CAD build for the part. Positions are in the model's coordinates, mm. Face numbers are marked on the shaded views. Give positions to 0.01 mm unless a question says otherwise; leave off trailing zeros. Loops run counter-clockwise (first coordinate to the right, second up) from the corner with the lowest first, then second, coordinate; pieces in that order, holes last. Notation, with made-up numbers: M 26.5,-36 L 73.5,-36 A4 ccw 73.5,-29 Z; hole C -27.75,52.5 d10. An arc over 180 degrees is marked long. Answer as CSV lines item,"result".
from build123d import *

# Parameters (mm, degrees)
SKETCH1_R                                           = 16.5
BOSS_EXTRUDE1_DEPTH                                 = 6
SKETCH25_R                                          = 10.25
BOSS_EXTRUDE2_DEPTH                                 = 2
SKETCH22_R                                          = 2.25
CUT_EXTRUDE1_DEPTH                                  = 46.38470183
CBORE_FOR_M2_HEX_SOCKET_HEAD_CAP_SCREW1_D           = 2.4
CBORE_FOR_M2_HEX_SOCKET_HEAD_CAP_SCREW1_CBORE_D     = 4.4
CBORE_FOR_M2_HEX_SOCKET_HEAD_CAP_SCREW1_CBORE_DEPTH = 2.4
CIRPATTERN1_COUNT                                   = 4
SKETCH26_R                                          = 4.5
CUT_EXTRUDE2_DEPTH                                  = 4.5


with BuildPart() as part:
    # Sketch1 → Boss-Extrude1 (new body)
    with BuildSketch(Plane(origin=(0, 0, 0), x_dir=(1, 0, 0), z_dir=(0, 1, 0))):
        with Locations(Location((0, 0, 0), (0, 0, 270))):
            Circle(SKETCH1_R)
    extrude(amount=-BOSS_EXTRUDE1_DEPTH)

    # Sketch25 → Boss-Extrude2 (add)
    with BuildSketch(Plane.XZ.offset(6)):
        with Locations(Location((0, 0, 0), (0, 0, 270))):
            Circle(SKETCH25_R)
    extrude(amount=BOSS_EXTRUDE2_DEPTH)

    # Sketch22 → Cut-Extrude1 (cut, through all)
    with BuildSketch(Plane(origin=(1.446175283, 0, 24.410951504), x_dir=(1, 0, 0), z_dir=(0, 1, 0))):
        with Locations(Location((-1.446175283, 35.724660003, 0), (0, 0, 270))):
            Circle(SKETCH22_R)
    cut_extrude1 = extrude(amount=-CUT_EXTRUDE1_DEPTH, mode=Mode.SUBTRACT)

    # Sketch3 → Cut-Revolve1 (revolve, cut)
    with BuildSketch(Plane(origin=(0, 0, -23.450692334), x_dir=(0, 0, -1), z_dir=(1, 0, 0))):
        Polygon((-12.136983835, 0), (-8.785226394, 0), (-9.185226394, -0.4), (-9.511983835, -2.725), (-9.511983835, -5.45), (-9.886983835, -5.825), (-12.136983835, -5.825), align=None)
    cut_revolve1 = revolve(axis=Axis((0, -5.825, -11.313708499), (0, 1, 0)), mode=Mode.SUBTRACT)

    # CBORE for M2 Hex Socket Head Cap Screw1 (through all)
    with Locations(Plane(origin=(0, 0, 0), x_dir=(1, 0, 0), z_dir=(0, 1, 0))):
        with Locations((5.656854249, 5.656854249)):
            cbore_for_m2_hex_socket_head_cap_screw1 = CounterBoreHole(CBORE_FOR_M2_HEX_SOCKET_HEAD_CAP_SCREW1_D / 2, CBORE_FOR_M2_HEX_SOCKET_HEAD_CAP_SCREW1_CBORE_D / 2, CBORE_FOR_M2_HEX_SOCKET_HEAD_CAP_SCREW1_CBORE_DEPTH)

    # CirPattern1: Cut-Extrude1, Cut-Revolve1, CBORE for M2 Hex Socket Head Cap Screw1 ×4 about axis
    cirpattern1_axis = Axis((0, 0, 0), (0, 1, 0))
    add([cut_extrude1.rotate(cirpattern1_axis, i * 360 / CIRPATTERN1_COUNT) for i in range(1, CIRPATTERN1_COUNT)], mode=Mode.SUBTRACT)
    add([cut_revolve1.rotate(cirpattern1_axis, i * 360 / CIRPATTERN1_COUNT) for i in range(1, CIRPATTERN1_COUNT)], mode=Mode.SUBTRACT)
    add([cbore_for_m2_hex_socket_head_cap_screw1.rotate(cirpattern1_axis, i * 360 / CIRPATTERN1_COUNT) for i in range(1, CIRPATTERN1_COUNT)], mode=Mode.SUBTRACT)

    # Sketch26 → Cut-Extrude2 (cut)
    with BuildSketch(Plane.XZ.offset(8)):
        with Locations(Location((0, 0, 0), (0, 0, 270))):
            Circle(SKETCH26_R)
    extrude(amount=-CUT_EXTRUDE2_DEPTH, mode=Mode.SUBTRACT)


solid = part.part
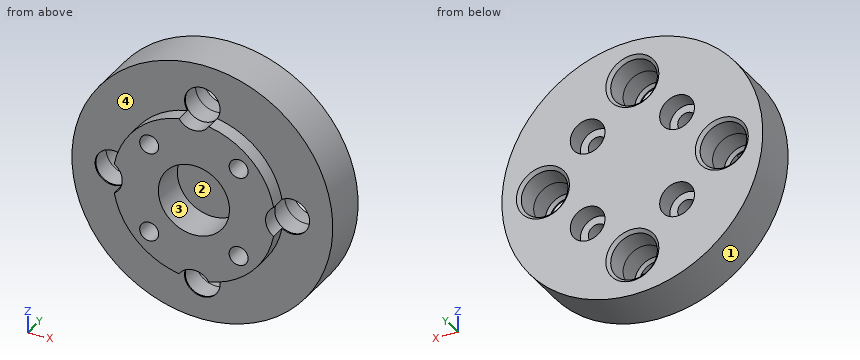
1) Flat gauge pins, fed straight in: pin 1 (2 mm diameter, centred on x = 11, z = 3.5, fed in from -Y); pin 2 (3 mm diameter, centred on x = -2, y = -2.5, fed in from -Z); pin 3 (3.5 mm diameter, centred on x = -5.66, z = 5.66, fed in from +Y); pin 4 (3.5 mm diameter, centred on x = 0, z = 11.31, fed in from +Y). Where does each tip first touch, or does it go through?
Answer below:
pin 1,"stops at y = -6"
pin 2,"stops at z = -16.49"
pin 3,"stops at y = -2.4"
pin 4,"passes through"
2) Mould opens along X. For the marked faces 1, 2, 3 and 4 say: +X half, -X half, draft (parallel to the pull), parting line (faces both ways), or undercut.
Answer below:
face 1,"parting line"
face 2,"undercut"
face 3,"undercut"
face 4,"draft"
3) Drill centre lines: line 1 (X direction, y = -4.5, z = -1.5); line 2 (Z direction, x = -6.5, y = -3); line 3 (Y direction, x = -3.5, z = 2.5). Where is each one in solid material? Low to high. Write a range as from..to.
Answer below:
line 1,"x = -16.43..-13.47, -9.16..-4.24, 4.24..9.16, 13.47..16.43"
line 2,"z = -15.17..-6.51, -4.8..4.8, 6.51..15.17"
line 3,"y = -3.5..0"
4) Band-saw the part on C-C on y = -6.75. Give the cut face in (x, z).
Answer below:
outline,"M -10.08,-1.88 A10.25 ccw -1.88,-10.08 A2.25 cw 1.88,-10.08 A10.25 ccw 10.08,-1.88 A2.25 cw 10.08,1.88 A10.25 ccw 1.88,10.08 A2.25 cw -1.88,10.08 A10.25 ccw -10.08,1.88 A2.25 cw Z; hole C -5.66,-5.66 d2.4; hole C -5.66,5.66 d2.4; hole C 0,0 d9; hole C 5.66,-5.66 d2.4; hole C 5.66,5.66 d2.4"
5) Band-saw the part on A-A on x = 0. Give the number of separate pieces and of enclosed holes in the cut face, and give its area (3 significant figures).
Answer below:
separate pieces,"3"
enclosed holes,"0"
area,"129 mm^2"
